Verification items for the finished model (mm, model axes). A direction names the side the tool comes from. Round coordinates to 2 decimals unless told otherwise and drop trailing zeros. Write each loop counter-clockwise with the first axis right and the second up, starting at its lowest first coordinate (ties: lowest second). Pieces come first, ordered by that corner, then holes. Notation, with made-up numbers: M -22,9 L 37,9 A26 ccw 37,40 Z; hole C 34.5,-16 d6. An arc over 180 degrees is marked long. Write each question's results on one line, items separated by ' | '.
from build123d import *

# Parameters (mm, degrees)
PAD_DEPTH       = 65
SKETCH052_R     = 1.625
POCKET_DEPTH    = 5
SKETCH053_R     = 2.875
POCKET001_DEPTH = 2
SKETCH054_R     = 1.35
POCKET002_DEPTH = 5
SKETCH055_W     = 20
SKETCH055_H     = 26
POCKET003_DEPTH = 2
POCKET004_DEPTH = 24.001
POCKET005_DEPTH = 45
SKETCH058_W     = 22.635606
SKETCH058_H     = 23.579969
PAD001_DEPTH    = 1.5
PAD002_DEPTH    = 1.5
POCKET006_DEPTH = 1.5
FILLET_R        = 15
FILLET001_R     = 48


with BuildPart() as part:
    # Sketch → Pad (new body)
    with BuildSketch(Plane.XZ):
        Polygon((0, -64), (0, 35), (-3, 35), (-3, -15), (-24, -15), (-24, -40), align=None)
    extrude(amount=PAD_DEPTH)

    # Sketch052 (on Face3 of Pad) → Pocket (cut)
    with BuildSketch(Plane(origin=(-3, 0, 0), x_dir=(0, 0, -1), z_dir=(-1, 0, 0))):
        with Locations((0, 5)):
            Circle(SKETCH052_R)
        with Locations((0, 50)):
            Circle(SKETCH052_R)
    extrude(amount=-POCKET_DEPTH, mode=Mode.SUBTRACT)

    # Sketch053 (on Face9 of Pocket) → Pocket001 (cut)
    with BuildSketch(Plane(origin=(-3, 0, 0), x_dir=(0, 0, -1), z_dir=(-1, 0, 0))):
        with Locations((0, 50)):
            Circle(SKETCH053_R)
        with Locations((0, 5)):
            Circle(SKETCH053_R)
    extrude(amount=-POCKET001_DEPTH, mode=Mode.SUBTRACT)

    # Sketch054 (on Face9 of Pocket001) → Pocket002 (cut)
    with BuildSketch(Plane(origin=(-3, 0, 0), x_dir=(0, 0, -1), z_dir=(-1, 0, 0))):
        with Locations((8.5, 62)):
            Circle(SKETCH054_R)
        with Locations((-30, 20)):
            Circle(SKETCH054_R)
    extrude(amount=-POCKET002_DEPTH, mode=Mode.SUBTRACT)

    # Sketch055 (on Face12 of Pocket002) → Pocket003 (cut)
    with BuildSketch(Plane(origin=(0, 0, -15), x_dir=(-1, 0, 0), z_dir=(0, 0, 1))):
        with Locations((13, 30)):
            Rectangle(SKETCH055_W, SKETCH055_H)
    extrude(amount=-POCKET003_DEPTH, mode=Mode.SUBTRACT)

    # Sketch056 (on Face10 of Pocket003) → Pocket004 (cut, through all)
    with BuildSketch(Plane(origin=(-24, 0, 0), x_dir=(0, 0, -1), z_dir=(-1, 0, 0))):
        Polygon((20, 65.935591), (65, 43), (65, 13), (20, -9.935591), (140.441742, -9.935591), (140.441742, 74.581261), align=None)
    extrude(amount=-POCKET004_DEPTH, mode=Mode.SUBTRACT)

    # Sketch057 (on Face3 of Pocket004) → Pocket005 (cut)
    with BuildSketch(Plane(origin=(0, 0, 0), x_dir=(1, 0, 0), z_dir=(0, 1, 0))):
        Polygon((-22.5, 16.5), (-1.5, 16.5), (-1.5, 60.37868), (-22.5, 39.37868), align=None)
    extrude(amount=-POCKET005_DEPTH, mode=Mode.SUBTRACT)

    # Sketch058 (on Face3 of Pocket005) → Pad001 (join)
    with BuildSketch(Plane(origin=(0, 0, 0), x_dir=(1, 0, 0), z_dir=(0, 1, 0))):
        with Locations((-12.082939, 27.703805)):
            Rectangle(SKETCH058_W, SKETCH058_H)
    extrude(amount=-PAD001_DEPTH)

    # Sketch059 (on Face2 of Pad001) → Pad002 (join)
    with BuildSketch(Plane(origin=(0, 15.978418, -8.143877), x_dir=(1, 0, 0), z_dir=(0, 0.890951, -0.4541))):
        Polygon((-0.967459, 35.017357), (-0.967459, 60.181422), (-23.34556, 35.017357), align=None)
    extrude(amount=-PAD002_DEPTH)

    # Sketch060 (on Face1 of Pad002) → Pocket006 (cut)
    with BuildSketch(Plane(origin=(0, 0, 0), x_dir=(0, 0, 1), z_dir=(1, 0, 0))):
        Polygon((-60.897689, 42.750073), (-52.897689, 44.883326), (-52.897689, 11.516028), (-60.897689, 12.750073), align=None)
    extrude(amount=-POCKET006_DEPTH, mode=Mode.SUBTRACT)

    # Fillet
    fillet_edges = [part.edges().sort_by_distance(p)[0] for p in [
        (-1.5, 0, 35),
    ]]
    fillet(fillet_edges, radius=FILLET_R)

    # Fillet001
    fillet001_edges = [part.edges().sort_by_distance(p)[0] for p in [
        (-1.5, -65, 35),
    ]]
    fillet(fillet001_edges, radius=FILLET001_R)


solid = part.part
1) Material ranges on line 1 (X direction, y = -32, z = -28); line 2 (Y direction, x = -0.3, z = 0) (3 decimals); line 3 (Z direction, x = -1.3, y = -20), recorded low to high. Write a range as [from, to].
Calculated:
line 1: x = [-24, -22.5], [-1.5, 0] | line 2: y = [-63.206, -51.625], [-48.375, -6.625], [-3.375, 0] | line 3: z = [-62.7, -60.9], [-52.9, 28.65], [31.35, 34.91]
2) Sectioned sample at A-A, the plane y = -5. Count the separate pieces of the cut face and the enclosed holes in it, and give its area (3 significant figures).
Calculated:
separate pieces: 2 | enclosed holes: 1 | area: 306 mm²
3) Sectioned sample at D-D, the plane z = -36. Record the cut outline in (x, y), and give its area (3 significant figures).
Calculated:
outline: M -24,-57.78 L 0,-57.78 L 0,0 L -24,0 Z; hole M -22.5,-45 L -1.5,-45 L -1.5,-1.5 L -22.5,-1.5 Z | area: 473 mm²
4) Sectioned sample at B-B, the plane z = 0. Record the cut outline in (x, y) (3 decimals), and give its area (3 significant figures).
Calculated:
outline: M -3,-63.206 L 0,-63.206 L 0,-51.625 L -1,-51.625 L -1,-52.875 L -3,-52.875 Z; M -3,-47.125 L -1,-47.125 L -1,-48.375 L 0,-48.375 L 0,-6.625 L -1,-6.625 L -1,-7.875 L -3,-7.875 Z; M -3,-2.125 L -1,-2.125 L -1,-3.375 L 0,-3.375 L 0,0 L -3,0 Z | area: 160 mm²
5) Access from +Z, -Z, +X, -X, +Y, -Y to the whole of each face (thin tool, end or side, straight path). Record for faces 1 (the flat face through (-1, -3, 0)), 2 (the flat face through (-13, -46, -15)), 3 (the flat face through (-13, -43, -16)), 4 (the flat face through (-22.5, -23, -28)).
Calculated:
face 1: -X | face 2: +Z, -X, +Y, -Y | face 3: +Z | face 4: none
6) Sectioned sample at C-C, the plane y = -20. Record the cut outline in (x, z).
Calculated:
outline: M -24,-40 L 0,-64 L 0,-60.9 L -1.5,-60.9 L -1.5,-60.38 L -22.5,-39.38 L -22.5,-17 L -23,-17 L -23,-15 L -24,-15 Z; M -3,-16.5 L -1.5,-16.5 L -1.5,-52.9 L 0,-52.9 L 0,28.65 L -3,28.65 Z; M -3,31.35 L 0,31.35 L 0,34.91 L -3,34.91 Z
7) Depth check by flat-ended pin: P1, Ø6.5, axis at x = -17.5, y = -34, coming from the +Z side; P2, Ø2, axis at x = -7, y = -16, coming from the -Z side; P3, Ø10, axis at x = -7.5, z = 24.5, coming from the +Y side. Enter the tip coordinate at first touch or a pass-through.
Calculated:
P1: stops at z = -41.13 | P2: stops at z = -58 | P3: stops at y = -0.18
8) Draft check along Z on faces 5 (the flat face through (-9.389, -6.737, -52.712)), 6 (the cylindrical face through (-2.01, -52.42, -1.55)), 7 (the flat face through (-12, -65, -18)). Enter one of: pulls with the +Z half, pulls with the -Z half, needs draft (parallel to the pull), parting line crosses it, or undercut.
Calculated:
face 5: pulls with the -Z half | face 6: undercut | face 7: needs draft
